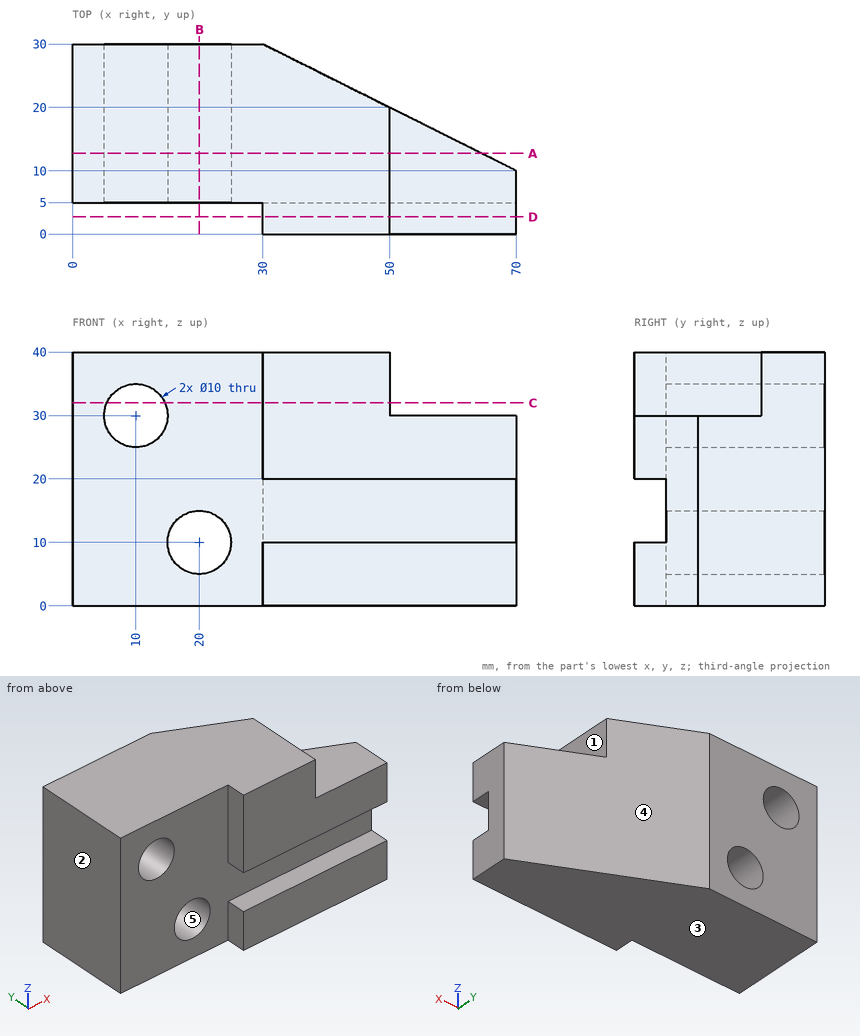
Study the drawing (mm; zero at the part's minimum x, y, z) and answer. A direction names the side the tool comes from. Round coordinates to 2 decimals unless told otherwise and drop trailing zeros. Order: outer loops, then holes, each group sorted by start corner. A loop starts at its lowest first (then second) coordinate and runs counter-clockwise, first axis right, second up. Notation, with made-up numbers: (82.5, 46) - (141.5, 46) arc R13 ccw to (141.5, 51) - close; hole circle Ø11 at (21.5, -2). An arc over 180 degrees is marked (long way). Use one line per item in the form item = value. Start each with the question number.
(1) For the marked faces 1 and 2, determine the directions among +Z, -Z, +X, -X, +Y, -Y from which every point of the face is accessible in a straight line to the end or side of a thin tool.
(2) The part is cut by section D-D (y = 2.75). Give the vertices of the cut face in (x, z).
(3) Find the intervals of material crossed by line 1 along Z through (x, y) = (10, 14.25); line 2 along Z through (x, y) = (20, 12.75); line 3 along X through (y, z) = (10, 10), in increasing order. Write a range as from..to.
(4) Flat-ended cylindrical pins translate along their axes: pin 1 Ø1.5 at (y, z) = (3.5, 7.5) entering from -X; pin 2 Ø5 at (x, y) = (44.5, 18) entering from -Z; pin 3 Ø2 at (x, z) = (60, 15) entering from +Y; pin 4 Ø2 at (x, z) = (13, 31.5) entering from +Y. Find the tip coordinate at first contact, or state that the pin passes through.
(5) The part is cut by section B-B (x = 20). Give the vertices of the cut face in (y, z).
(6) The part is cut by section C-C (z = 32). Give the vertices of the cut face in (x, y).
(7) Determine the mould class of the marked faces 3, 4 and 5 for opening direction Z: +Z half, -Z half, draft (parallel to the pull), parting line (faces both ways), or undercut.
(8) The part is cut by section A-A (y = 12.75). Give the vertices of the cut face in (x, z).
Checked values:
q1.face_1 = +Z, +X, +Y, -Y
q1.face_2 = +Z, -Z, -X, +Y, -Y
q2.outline = (30, 0) - (70, 0) - (70, 10) - (30, 10) - close; (30, 20) - (70, 20) - (70, 30) - (50, 30) - (50, 40) - (30, 40) - close
q3.line_1 = 0..25, 35..40
q3.line_2 = 0..5, 15..40
q3.line_3 = 0..15, 25..70
q4.pin_1 = 30
q4.pin_2 = 0
q4.pin_3 = 15.5
q4.pin_4 = through
q5.outline = (5, 0) - (30, 0) - (30, 5) - (5, 5) - close; (5, 15) - (30, 15) - (30, 40) - (5, 40) - close
q6.outline = (0, 5) - (5.42, 5) - (5.42, 30) - (0, 30) - close; (14.58, 5) - (30, 5) - (30, 0) - (50, 0) - (50, 20) - (30, 30) - (14.58, 30) - close
q7.face_3 = -Z half
q7.face_4 = draft
q7.face_5 = undercut
q8.outline = (0, 0) - (64.5, 0) - (64.5, 30) - (50, 30) - (50, 40) - (0, 40) - close; hole circle Ø10 at (10, 30); hole circle Ø10 at (20, 10)
